Read the model definition and answer for the solid it produces. Units are mm, in the model's axes. A direction names the side the tool comes from. Give positions to 0.01 mm unless a question says otherwise; leave off trailing zeros. Loops run counter-clockwise (first coordinate to the right, second up) from the corner with the lowest first, then second, coordinate; pieces in that order, holes last. Notation, with made-up numbers: (-35.75, 17.25) -> (-29.75, 17.25) arc R25 cw to (-29.75, 32.25) -> close; hole circle Ø8 at (63, 11). An arc over 180 degrees is marked (long way). Answer as CSV lines item,"result". Start each with the question number.
```python
from build123d import *

# Parameters (mm, degrees)
F0_R     = 2.5908
F1_DEPTH = 4.572
F2_DEPTH = 12.446
F3_R     = 2.0193
F4_DEPTH = 50.8


with BuildPart() as f1:
    # F0 (on Front) → F1 (new body)
    with BuildSketch(Plane.XZ):
        with BuildLine():
            Line((26.4033, 0), (28.575, 0))
            ThreePointArc((28.575, 0), (20.2055762724, 20.2055762724), (0, 28.575))
            Line((0, 28.575), (0, 12.1666))
            ThreePointArc((0, 12.1666), (8.603085364, 8.603085364), (12.1666, 0))
            Line((12.1666, 0), (21.2217, 0))
            ThreePointArc((21.2217, 0), (23.8125, 2.5908), (26.4033, 0))
        make_face()
        with Locations((11.7190584855, 20.7291780943)):
            Circle(F0_R, mode=Mode.SUBTRACT)
        with BuildLine():
            ThreePointArc((0, -28.575), (20.2055762724, -20.2055762724), (28.575, 0))
            Line((28.575, 0), (26.4033, 0))
            ThreePointArc((26.4033, 0), (23.8125, -2.5908), (21.2217, 0))
            Line((21.2217, 0), (12.1666, 0))
            ThreePointArc((12.1666, 0), (9.1104172738, -8.0638981055), (1.4772615395, -12.0765828736))
            ThreePointArc((1.4772615395, -12.0765828736), (0.7400008006, -12.144074867), (0, -12.1666))
            Line((0, -12.1666), (0, -28.575))
        make_face()
        with Locations((11.7190584855, -20.7291780943)):
            Circle(F0_R, mode=Mode.SUBTRACT)
        with BuildLine():
            Line((0, 12.1666), (0, 28.575))
            ThreePointArc((0, 28.575), (-20.2055762724, 20.2055762724), (-28.575, 0))
            Line((-28.575, 0), (-26.4033, 0))
            ThreePointArc((-26.4033, 0), (-23.8125, 2.5908), (-21.2217, 0))
            Line((-21.2217, 0), (-12.1666, 0))
            ThreePointArc((-12.1666, 0), (-8.603085364, 8.603085364), (0, 12.1666))
        make_face()
        with Locations((-14.0022196536, 19.260659413)):
            Circle(F0_R, mode=Mode.SUBTRACT)
        with BuildLine():
            ThreePointArc((-28.575, 0), (-20.2055762724, -20.2055762724), (0, -28.575))
            Line((0, -28.575), (0, -12.1666))
            ThreePointArc((0, -12.1666), (-0.7613836332, -12.1427530043), (-1.5197825851, -12.0713054992))
            ThreePointArc((-1.5197825851, -12.0713054992), (-9.1246025217, -8.0478434615), (-12.1666, 0))
            Line((-12.1666, 0), (-21.2217, 0))
            ThreePointArc((-21.2217, 0), (-23.8125, -2.5908), (-26.4033, 0))
            Line((-26.4033, 0), (-28.575, 0))
        make_face()
        with BuildLine():
            ThreePointArc((-13.8432016041, -21.9729224119), (-15.6621403898, -17.5467676407), (-11.2427748724, -19.3821402972))
            ThreePointArc((-11.2427748724, -19.3821402972), (-12.0050093549, -21.2175129537), (-13.8432016041, -21.9729224119))
        make_face(mode=Mode.SUBTRACT)
    extrude(amount=F1_DEPTH)

    # F0 (on Front) → F2 (join)
    with BuildSketch(Plane.XZ):
        with BuildLine():
            Line((-3.72745, 0), (-12.1666, 0))
            ThreePointArc((-12.1666, 0), (-9.1246025217, -8.0478434615), (-1.5197825851, -12.0713054992))
            Line((-1.5197825851, -12.0713054992), (-1.5197825851, -1.9539885713))
            Line((-1.5197825851, -1.9539885713), (-3.1742419829, -1.9539885713))
            ThreePointArc((-3.1742419829, -1.9539885713), (-3.586482384, -1.0153952982), (-3.72745, 0))
        make_face()
        with BuildLine():
            ThreePointArc((1.4772615395, -12.0765828736), (9.1104172738, -8.0638981055), (12.1666, 0))
            Line((12.1666, 0), (3.72745, 0))
            ThreePointArc((3.72745, 0), (3.586482384, -1.0153952982), (3.1742419829, -1.9539885713))
            Line((3.1742419829, -1.9539885713), (1.4772615395, -1.9539885713))
            Line((1.4772615395, -1.9539885713), (1.4772615395, -12.0765828736))
        make_face()
        with BuildLine():
            ThreePointArc((12.1666, 0), (8.603085364, 8.603085364), (0, 12.1666))
            Line((0, 12.1666), (0, 2.3218799357))
            Line((0, 2.3218799357), (2.9159487421, 2.3218799357))
            ThreePointArc((2.9159487421, 2.3218799357), (3.5187310668, 1.2298029036), (3.72745, 0))
            Line((3.72745, 0), (12.1666, 0))
        make_face()
        with BuildLine():
            Line((0, 2.3218799357), (0, 12.1666))
            ThreePointArc((0, 12.1666), (-8.603085364, 8.603085364), (-12.1666, 0))
            Line((-12.1666, 0), (-3.72745, 0))
            ThreePointArc((-3.72745, 0), (-3.5187310668, 1.2298029036), (-2.9159487421, 2.3218799357))
            Line((-2.9159487421, 2.3218799357), (0, 2.3218799357))
        make_face()
        with BuildLine():
            Line((0, -1.9539885713), (0, -12.1666))
            ThreePointArc((0, -12.1666), (0.7400008006, -12.144074867), (1.4772615395, -12.0765828736))
            Line((1.4772615395, -12.0765828736), (1.4772615395, -1.9539885713))
            Line((1.4772615395, -1.9539885713), (0, -1.9539885713))
        make_face()
        with BuildLine():
            ThreePointArc((-1.5197825851, -12.0713054992), (-0.7613836332, -12.1427530043), (0, -12.1666))
            Line((0, -12.1666), (0, -1.9539885713))
            Line((0, -1.9539885713), (-1.5197825851, -1.9539885713))
            Line((-1.5197825851, -1.9539885713), (-1.5197825851, -12.0713054992))
        make_face()
    extrude(amount=F2_DEPTH)

    # F3 (on Top) → F4 (cut)
    with BuildSketch(Plane.XY):
        with Locations((0, -8.1789378586)):
            Circle(F3_R)
    extrude(amount=F4_DEPTH, mode=Mode.SUBTRACT)


solid = f1.part
```
(1) Find section D-D on z = -1. Write down the section's boundary in (x, y), then the cut area to 3 significant figures.
(2) Find section C-C on y = -3.5. Give the number of separate pieces and of enclosed holes in the cut face, then the cut area to 3 significant figures.
(3) Find section A-A on x = -13. Write down the section's boundary in (y, z), then the cut area to 3 significant figures.
(4) The mould has two halves that part along Y. Classify faces 1 (the face through (6, 0, 0)), 2 (the face through (-0.44, -10.15, 7.18)), 3 (the face through (26.284, -2.254, -0.778)), 4 (the face through (0, -12.446, -3)): pulls with the +Y half, pulls with the -Y half, needs draft (parallel to the pull), parting line crosses it, or undercut.
(5) Find the intervals of material crossed by line 1 along Y through (x, z) = (3, 22.5); line 2 along Z through (x, y) = (16.5, -1); line 3 along Z through (x, y) = (11, -0.5), in increasing order. Write a range as from..to.
(6) Each of these flat-tipped pins is pushed along its axis until it touches: P1, Ø2, axis at x = 7, y = -7.5, coming from the +Z side; P2, Ø6.5, axis at x = -13.83, z = -19.38, coming from the -Y side; P3, Ø4.5, axis at x = 0, y = -8.18, coming from the -Z side; P4, Ø4, axis at x = 11.72, z = -20.73, coming from the +Y side. Where does it stop, or does it pass through?
(7) Find section B-B on x = -23.5. Write down the section's boundary in (y, z).
(8) A tool of negligible diameter and unlimited length cuts with its end or side. For faces 5 (the face through (12, -4.572, -6)), 6 (the face through (0, -6, -1.954)), from which of +Z, -Z, +X, -X, +Y, -Y can it reach the whole face along a straight path? Write none if from no direction.
Answer block:
1,outline,"(-28.56, -4.57) -> (-26.2, -4.57) -> (-26.2, 0) -> (-28.56, 0) -> close; (-21.42, -4.57) -> (-12.13, -4.57) -> (-12.13, -12.45) -> (-3.59, -12.45) -> (-3.59, 0) -> (-21.42, 0) -> close; (3.59, -12.45) -> (12.13, -12.45) -> (12.13, -4.57) -> (21.42, -4.57) -> (21.42, 0) -> (3.59, 0) -> close; (26.2, -4.57) -> (28.56, -4.57) -> (28.56, 0) -> (26.2, 0) -> close"
1,area,"319 mm2"
2,separate pieces,"1"
2,enclosed holes,"7"
2,area,"2,410 mm2"
3,outline,"(-4.57, -25.45) -> (0, -25.45) -> (0, -21.84) -> (-4.57, -21.84) -> close; (-4.57, -16.93) -> (0, -16.93) -> (0, 16.87) -> (-4.57, 16.87) -> close; (-4.57, 21.65) -> (0, 21.65) -> (0, 25.45) -> (-4.57, 25.45) -> close"
3,area,"188 mm2"
4,face 1,"pulls with the +Y half"
4,face 2,"undercut"
4,face 3,"needs draft"
4,face 4,"pulls with the -Y half"
5,line 1,"y = -4.57..0"
5,line 2,"z = -23.33..23.33"
5,line 3,"z = -26.37..-23.22, -18.24..18.24, 23.22..26.37"
6,P1,"stops at z = 10.58"
6,P2,"stops at y = -4.57"
6,P3,"stops at z = -12.17"
6,P4,"passes through"
7,outline,"(-4.57, -16.26) -> (0, -16.26) -> (0, -2.57) -> (-4.57, -2.57) -> close; (-4.57, 2.57) -> (0, 2.57) -> (0, 16.26) -> (-4.57, 16.26) -> close"
8,face 5,"-Y"
8,face 6,"+Y, -Y"
